from build123d import *

# Parameters (mm, degrees)
F0_R     = 7.95
F1_DEPTH = 3
F2_R     = 8.95
F3_DEPTH = 3.5
F4_R     = 7.95
F5_DEPTH = 3
F6_R     = 1.4204913212
F7_DEPTH = 9.501
F8_R     = 6.9107531966
F8_R_2   = 3
F8_R_3   = 1.05
F9_DEPTH = 5


with BuildPart() as f1:
    # F0 (on Top) → F1 (new body)
    with BuildSketch(Plane.XY):
        Circle(F0_R)
    extrude(amount=F1_DEPTH)

    # F2 (on face) → F3 (join)
    with BuildSketch(Plane.XY.offset(3)):
        Circle(F2_R)
    extrude(amount=F3_DEPTH)

    # F4 (on face) → F5 (join)
    with BuildSketch(Plane.XY.offset(6.5)):
        Circle(F4_R)
    extrude(amount=F5_DEPTH)

    # F6 (on face) → F7 (cut, through all)
    with BuildSketch(Plane.XY.offset(9.5)):
        with Locations((-0.869839613, 5.4209182347)):
            Circle(F6_R)
        with Locations((-4.2597330966, -3.4637623194)):
            Circle(F6_R)
        with Locations((5.1295727096, -1.9571559153)):
            Circle(F6_R)
    extrude(amount=-F7_DEPTH, mode=Mode.SUBTRACT)

    # F8 (on face) → F9 (cut)
    with BuildSketch(Plane(origin=(0, 0, 0), x_dir=(1, 0, 0), z_dir=(0, 0, -1))):
        Circle(F8_R)
        Circle(F8_R_2, mode=Mode.SUBTRACT)
        Circle(F8_R_3)
    extrude(amount=-F9_DEPTH, mode=Mode.SUBTRACT)


solid = f1.part
Model file for the job. Use its own axes, mm. A direction names the side the tool comes from. Round coordinates to 2 decimals unless told otherwise and drop trailing zeros. Order: outer loops, then holes, each group sorted by start corner. A loop starts at its lowest first (then second) coordinate and runs counter-clockwise, first axis right, second up.
(1) Band-saw the part on A-A (x = 0.25). List the corners of the cut face in (y, z).
(2) Drill centre lines: line 1 (Y direction, x = 0, z = 2.05); line 2 (Y direction, x = 0, z = 3.5); line 3 (Y direction, x = -1.75, z = 2.5) (1 decimal). Where is each one in solid material? Low to high.
(3) Band-saw the part on B-B (y = 0). List the corners of the cut face in (x, z).
(4) Band-saw the part on C-C (z = 4). List the corners of the cut face in (x, y).
(5) 3-axis set-ups, long thin cutter, end or side, ignore diameter. For faces 1 (the face through (1, -0.32, 2.46)), 2 (the face through (-1.4, 8, 6.5)), 3 (the face through (0, 0, 9.5)): which of +Z, -Z, +X, -X, +Y, -Y reach the whole face in a straight line?
(6) Pin check, flat tips, straight feed: pin 1 (1 mm diameter, centred on x = -4.5, z = 7.5, fed in from -Y); pin 2 (1 mm diameter, centred on x = -1.5, z = 1, fed in from +Y); pin 3 (1 mm diameter, centred on x = 0, y = 0, fed in from -Z); pin 4 (2.5 mm diameter, centred on x = 5.13, y = -1.96, fed in from +Z). Stop position of each tip, or through.
(7) Pull direction X, two halves, no side cores. Call faces 4 (the face through (-1.4, 8, 3)), 5 (the face through (-1.72, -7.76, 7.98)), 6 (the face through (6.484, -1.53, 7.281)): released by +X, released by -X, zero draft, split by the parting line, or undercut.
(8) Band-saw the part on D-D (y = -3.75). List the corners of the cut face in (x, z).
Verdict:
1. outline: (-8.95, 3) - (-7.95, 3) - (-7.95, 0) - (-6.91, 0) - (-6.91, 5) - (-2.99, 5) - (-2.99, 0) - (-1.02, 0) - (-1.02, 5) - (1.02, 5) - (1.02, 0) - (2.99, 0) - (2.99, 5) - (4.55, 5) - (4.55, 9.5) - (-7.95, 9.5) - (-7.95, 6.5) - (-8.95, 6.5) - close; (6.29, 5) - (6.91, 5) - (6.91, 0) - (7.95, 0) - (7.95, 3) - (8.95, 3) - (8.95, 6.5) - (7.95, 6.5) - (7.95, 9.5) - (6.29, 9.5) - close
2. line 1: y = -7.95 to -6.91, -3 to -1.05, 1.05 to 3, 6.91 to 7.95
2. line 2: y = -8.95 to -6.91, -3 to -1.05, 1.05 to 3, 6.91 to 8.95
2. line 3: y = -7.8 to -6.7, -2.4 to 2.4, 6.7 to 7.8
3. outline: (-8.95, 3) - (-7.95, 3) - (-7.95, 0) - (-6.91, 0) - (-6.91, 5) - (-3, 5) - (-3, 0) - (-1.05, 0) - (-1.05, 5) - (1.05, 5) - (1.05, 0) - (3, 0) - (3, 5) - (6.91, 5) - (6.91, 0) - (7.95, 0) - (7.95, 3) - (8.95, 3) - (8.95, 6.5) - (7.95, 6.5) - (7.95, 9.5) - (-7.95, 9.5) - (-7.95, 6.5) - (-8.95, 6.5) - close
4. outline: circle Ø17.9 at (0, 0); circle Ø6 at (0, 0); hole circle Ø13.82 at (0, 0); hole circle Ø2.1 at (0, 0)
5. face 1: -Z
5. face 2: +Z
5. face 3: +Z, +X, -X, +Y, -Y
6. pin 1: stops at y = -6.87
6. pin 2: stops at y = 7.89
6. pin 3: stops at z = 5
6. pin 4: passes through
7. face 4: zero draft
7. face 5: split by the parting line
7. face 6: undercut
8. outline: (-8.13, 3) - (-7.01, 3) - (-7.01, 0) - (-5.8, 0) - (-5.8, 5) - (-5.65, 5) - (-5.65, 9.5) - (-7.01, 9.5) - (-7.01, 6.5) - (-8.13, 6.5) - close; (-2.87, 5) - (5.8, 5) - (5.8, 0) - (7.01, 0) - (7.01, 3) - (8.13, 3) - (8.13, 6.5) - (7.01, 6.5) - (7.01, 9.5) - (-2.87, 9.5) - close
